The listing builds one solid part. Answer for the finished solid, in the listing's coordinates (mm). Face numbers are marked on the shaded views. A direction names the side the tool comes from. Round coordinates to 2 decimals unless told otherwise and drop trailing zeros. Write each loop counter-clockwise with the first axis right and the second up, starting at its lowest first coordinate (ties: lowest second). Pieces come first, ordered by that corner, then holes. Notation, with made-up numbers: (21, -24.5) - (53, -24.5) arc R27 cw to (53, 10.5) - close; hole circle Ø10 at (-15.75, 14). An arc over 180 degrees is marked (long way). Use a Markdown table: item, result. Add a question column.
1) A tool of negligible diameter and unlimited length cuts with its end or side. For the marked faces 1, 2, 3, 4 and 5, from which of +Z, -Z, +X, -X, +Y, -Y can it reach the whole face along a straight path? Write none if from no direction.
2) Find the intervals of material crossed by probe 1 along X at (y, z) = (3.25, -249.5); probe 2 along Z at (x, y) = (126, 5); probe 3 along X at (y, z) = (4.75, -46), in increasing order. Write a range as from..to.
3) A cutting plane is placed at D-D (y = 4). State how many separate pieces and enclosed holes the cut face has, then the cut area to 3 significant figures.
4) Each of these flat-tipped pins is pushed along its axis until it touches: P1, Ø0.8, axis at y = 7, z = -8.5, coming from the -X side; P2, Ø5, axis at y = 3, z = -411.5, coming from the -X side; P3, Ø10, axis at x = 2, z = -379, coming from the +Y side. Where does it stop, or does it pass through?
5) A cutting plane is placed at C-C (z = -301). Give the vertices of the cut face in (x, y).
6) A cutting plane is placed at A-A (z = -14). Give the vertices of the cut face in (x, y), then the cut area to 3 significant figures.
7) A cutting plane is placed at B-B (x = 57.15). Give the vertices of the cut face in (y, z), then the cut area to 3 significant figures.
8) Determine the mould class of the marked faces 6 and 7 for opening direction X: +X half, -X half, draft (parallel to the pull), parting line (faces both ways), or undercut.
```python
from build123d import *

# Parameters (mm, degrees)
SKETCH2_W           = 457.2
SKETCH2_H           = 457.2
SKETCH2_W_2         = 12.7
SKETCH2_H_2         = 12.7
SKETCH2_W_3         = 50.8
SKETCH2_H_3         = 177.8
SKETCH2_W_4         = 76.2
SKETCH2_H_4         = 76.2
BOSS_EXTRUDE1_DEPTH = 6.35
SKETCH3_W           = 2.54
SKETCH3_H           = 25.4
BOSS_EXTRUDE2_DEPTH = 2.54


with BuildPart() as part:
    # Sketch2 → Boss-Extrude1 (new body)
    with BuildSketch(Plane(origin=(0, 0, 0), x_dir=(1, 0, 0), z_dir=(0, 1, 0))):
        with Locations((228.6, 228.6)):
            Rectangle(SKETCH2_W, SKETCH2_H)
        with BuildLine():
            Line((31.75, 438.15), (31.75, 387.35))
            ThreePointArc((31.75, 387.35), (19.05, 374.65), (6.35, 387.35))
            Line((6.35, 387.35), (6.35, 438.15))
            ThreePointArc((6.35, 438.15), (19.05, 450.85), (31.75, 438.15))
        make_face(mode=Mode.SUBTRACT)
        with BuildLine():
            Line((69.85, 438.15), (69.85, 387.35))
            ThreePointArc((69.85, 387.35), (57.15, 374.65), (44.45, 387.35))
            Line((44.45, 387.35), (44.45, 438.15))
            ThreePointArc((44.45, 438.15), (57.15, 450.85), (69.85, 438.15))
        make_face(mode=Mode.SUBTRACT)
        with BuildLine():
            Line((425.45, 438.15), (425.45, 387.35))
            ThreePointArc((425.45, 387.35), (438.15, 374.65), (450.85, 387.35))
            Line((450.85, 387.35), (450.85, 438.15))
            ThreePointArc((450.85, 438.15), (438.15, 450.85), (425.45, 438.15))
        make_face(mode=Mode.SUBTRACT)
        with BuildLine():
            Line((387.35, 438.15), (387.35, 387.35))
            ThreePointArc((387.35, 387.35), (400.05, 374.65), (412.75, 387.35))
            Line((412.75, 387.35), (412.75, 438.15))
            ThreePointArc((412.75, 438.15), (400.05, 450.85), (387.35, 438.15))
        make_face(mode=Mode.SUBTRACT)
        with Locations((330.2, 412.75)):
            Rectangle(SKETCH2_W_2, SKETCH2_H_2, mode=Mode.SUBTRACT)
        with Locations((127, 292.1)):
            Rectangle(SKETCH2_W_3, SKETCH2_H_3, mode=Mode.SUBTRACT)
        with Locations((127, 412.75)):
            Rectangle(SKETCH2_W_2, SKETCH2_H_2, mode=Mode.SUBTRACT)
        with Locations((330.2, 292.1)):
            Rectangle(SKETCH2_W_3, SKETCH2_H_3, mode=Mode.SUBTRACT)
        with Locations((412.75, 44.45)):
            Rectangle(SKETCH2_W_4, SKETCH2_H_4, mode=Mode.SUBTRACT)
        with Locations((44.45, 44.45)):
            Rectangle(SKETCH2_W_4, SKETCH2_H_4, mode=Mode.SUBTRACT)
    extrude(amount=BOSS_EXTRUDE1_DEPTH)

    # Sketch3 → Boss-Extrude2 (add)
    with BuildSketch(Plane(origin=(0, 6.35, 0), x_dir=(1, 0, 0), z_dir=(0, 1, 0))):
        with BuildLine():
            Line((120.65, 411.48), (-19.05, 411.48))
            Line((-19.05, 411.48), (-19.05, 285.75))
            ThreePointArc((-19.05, 285.75), (-44.45, 260.35), (-69.85, 285.75))
            Line((-69.85, 285.75), (-69.85, 539.75))
            ThreePointArc((-69.85, 539.75), (-44.45, 565.15), (-19.05, 539.75))
            Line((-19.05, 539.75), (-19.05, 414.02))
            Line((-19.05, 414.02), (120.65, 414.02))
            Line((120.65, 414.02), (120.65, 411.48))
        make_face()
        with Locations((127, 393.7)):
            Rectangle(SKETCH3_W, SKETCH3_H)
        with Locations((330.2, 393.7)):
            Rectangle(SKETCH3_W, SKETCH3_H)
        with BuildLine():
            Line((336.55, 411.48), (336.55, 414.02))
            Line((336.55, 414.02), (476.25, 414.02))
            Line((476.25, 414.02), (476.25, 539.75))
            ThreePointArc((476.25, 539.75), (501.65, 565.15), (527.05, 539.75))
            Line((527.05, 539.75), (527.05, 285.75))
            ThreePointArc((527.05, 285.75), (501.65, 260.35), (476.25, 285.75))
            Line((476.25, 285.75), (476.25, 411.48))
            Line((476.25, 411.48), (336.55, 411.48))
        make_face()
        with BuildLine():
            Line((69.85, 139.7), (69.85, -50.8))
            ThreePointArc((69.85, -50.8), (44.45, -76.2), (19.05, -50.8))
            Line((19.05, -50.8), (19.05, 139.7))
            ThreePointArc((19.05, 139.7), (44.45, 165.1), (69.85, 139.7))
        make_face()
        with BuildLine():
            Line((387.35, 139.7), (387.35, -50.8))
            ThreePointArc((387.35, -50.8), (412.75, -76.2), (438.15, -50.8))
            Line((438.15, -50.8), (438.15, 139.7))
            ThreePointArc((438.15, 139.7), (412.75, 165.1), (387.35, 139.7))
        make_face()
    extrude(amount=BOSS_EXTRUDE2_DEPTH)


solid = part.part
```
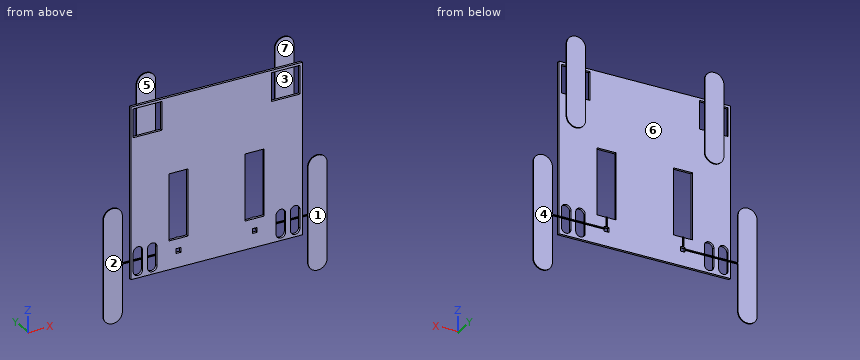
Entries:
| question | item | result |
|---|---|---|
| 1 | face 1 | +Z, -Z, +X, -Y |
| 1 | face 2 | +Z, -Z, -X, -Y |
| 1 | face 3 | -Y |
| 1 | face 4 | +Z, -Z, +X, -X, +Y |
| 1 | face 5 | +Z, +X, -X, -Y |
| 2 | probe 1 | x = 0..101.6, 152.4..304.8, 355.6..457.2 |
| 2 | probe 2 | z = -457.2..-419.1, -406.4..-381, -203.2..0 |
| 2 | probe 3 | x = 0..6.35, 82.55..374.65, 450.85..457.2 |
| 3 | separate pieces | 1 |
| 3 | enclosed holes | 10 |
| 3 | area | 172,000 mm² |
| 4 | P1 | stops at x = 19.05 |
| 4 | P2 | stops at x = 0 |
| 4 | P3 | stops at y = 6.35 |
| 5 | outline | (-69.85, 6.35) - (-19.05, 6.35) - (-19.05, 8.89) - (-69.85, 8.89) - close; (0, 0) - (101.6, 0) - (101.6, 6.35) - (0, 6.35) - close; (152.4, 0) - (304.8, 0) - (304.8, 6.35) - (152.4, 6.35) - close; (355.6, 0) - (457.2, 0) - (457.2, 6.35) - (355.6, 6.35) - close; (476.25, 6.35) - (527.05, 6.35) - (527.05, 8.89) - (476.25, 8.89) - close |
| 6 | outline | (0, 0) - (6.35, 0) - (6.35, 6.35) - (0, 6.35) - close; (19.05, 6.35) - (69.85, 6.35) - (69.85, 8.89) - (19.05, 8.89) - close; (82.55, 0) - (374.65, 0) - (374.65, 6.35) - (82.55, 6.35) - close; (387.35, 6.35) - (438.15, 6.35) - (438.15, 8.89) - (387.35, 8.89) - close; (450.85, 0) - (457.2, 0) - (457.2, 6.35) - (450.85, 6.35) - close |
| 6 | area | 2,190 mm² |
| 7 | outline | (0, -457.2) - (6.35, -457.2) - (6.35, -450.85) - (0, -450.85) - close; (0, -374.65) - (6.35, -374.65) - (6.35, -161.7) - (8.89, -161.7) - (8.89, 72.8) - (6.35, 72.8) - (6.35, 0) - (0, 0) - (0, -6.35) - (6.35, -6.35) - (6.35, -82.55) - (0, -82.55) - close; (6.35, -414.02) - (8.89, -414.02) - (8.89, -411.48) - (6.35, -411.48) - close |
| 7 | area | 2,540 mm² |
| 8 | face 6 | undercut |
| 8 | face 7 | draft |
